```python
from build123d import *

# Parameters (mm, degrees)
CUT_EXTRUDE_1_DEPTH = 0.55


with BuildPart() as part:
    # 草图1 → 旋转1 (revolve)
    with BuildSketch(Plane.XY, mode=Mode.PRIVATE) as revolve_1_sk:
        Polygon((12, 1.6), (11.6, 2), (0, 2), (0, 0), (12, 0), align=None)
        with BuildLine():
            Line((-0.11, 4), (-0.99, 4))
            ThreePointArc((-0.99, 4), (-1.067781746, 3.967781746), (-1.1, 3.89))
            Line((-1.1, 3.89), (-1.1, 0))
            Line((-1.1, 0), (0, 0))
            Line((0, 0), (0, 3.89))
            ThreePointArc((0, 3.89), (-0.032218254, 3.967781746), (-0.11, 4))
        make_face()
    revolve(revolve_1_sk.sketch.rotate(Axis((0, 0, 0), (1, 0, 0)), 90), axis=Axis((0, 0, 0), (1, 0, 0)))

    # 草图2 → 切除-拉伸1 (cut)
    with BuildSketch(Plane.ZY.offset(1.1)):
        Polygon((1.25, -0.721687836), (1.25, 0.721687836), (0, 1.443375673), (-1.25, 0.721687836), (-1.25, -0.721687836), (0, -1.443375673), align=None)
    extrude(amount=-CUT_EXTRUDE_1_DEPTH, mode=Mode.SUBTRACT)


solid = part.part
```
CAD build for the part. Positions are in the model's coordinates, mm. A direction names the side the tool comes from. Round coordinates to 2 decimals unless told otherwise and drop trailing zeros. Order: outer loops, then holes, each group sorted by start corner. A loop starts at its lowest first (then second) coordinate and runs counter-clockwise, first axis right, second up.
Item 1: Saw through at B-B on x = 10.75. Write the cut outline in (y, z), then the cut area to 3 significant figures.
Item 2: Tool access for faces 4 (the face through (0, -1, 2)), 5 (the face through (-0.556, 3.905, -0.867)): list every direction of +Z, -Z, +X, -X, +Y, -Y with a clear straight run to the whole face (end or side of a thin tool).
Item 3: Mould opens along Z. For faces 1 (the face through (-0.55, 0, 0)), 2 (the face through (12, 0, 0)), 3 (the face through (6, 2, 0)) say: pulls with the +Z half, pulls with the -Z half, needs draft (parallel to the pull), parting line crosses it, or undercut.
Item 4: Saw through at A-A on y = 0. Write the cut outline in (x, z), then the cut area to 3 significant figures.
Item 5: Probe line 1 along X through (y, z) = (-3, 0); line 2 along Y through (x, z) = (3.25, 0); line 3 along Z through (x, y) = (4.25, -1.25). List the from-to ranges inside material, lowest first.
Item 6: Pin check, flat tips, straight feed: pin 1 (1 mm diameter, centred on x = 1.5, z = 0, fed in from -Y); pin 2 (1.5 mm diameter, centred on x = 6, z = 1.5, fed in from -Y); pin 3 (1 mm diameter, centred on x = 5.5, z = -2, fed in from -Y). Stop position of each tip, or through.
Reported:
1. outline: circle Ø4 at (0, 0)
1. area: 12.6 mm2
2. face 4: +X
2. face 5: +X, -X
3. face 1: undercut
3. face 2: needs draft
3. face 3: parting line crosses it
4. outline: (-1.1, -3.89) arc R0.11 ccw to (-0.99, -4) - (-0.11, -4) arc R0.11 ccw to (0, -3.89) - (0, -2) - (11.6, -2) - (12, -1.6) - (12, 1.6) - (11.6, 2) - (0, 2) - (0, 3.89) arc R0.11 ccw to (-0.11, 4) - (-0.99, 4) arc R0.11 ccw to (-1.1, 3.89) - (-1.1, 1.25) - (-0.55, 1.25) - (-0.55, -1.25) - (-1.1, -1.25) - close
4. area: 55.3 mm2
5. line 1: x = -1.1 to 0
5. line 2: y = -2 to 2
5. line 3: z = -1.56 to 1.56
6. pin 1: stops at y = -2
6. pin 2: stops at y = -1.85
6. pin 3: stops at y = -1.32
